Verification items for the finished model (mm, model axes). Face numbers are marked on the shaded views. A direction names the side the tool comes from. Coordinates: 2 decimals unless noted, no trailing zeros. Order: outer loops, then holes, each group sorted by start corner. A loop starts at its lowest first (then second) coordinate and runs counter-clockwise, first axis right, second up.
Q1. Draft check along X on the marked faces 1 and 2. Enter one of: pulls with the +X half, pulls with the -X half, needs draft (parallel to the pull), parting line crosses it, or undercut.
Q2. Depth check by flat-ended pin: P1, Ø2.5, axis at x = 23, y = 20.5, coming from the +Z side. Enter the tip coordinate at first touch or a pass-through.
Q3. Cross-section at D-D, the plane x = -14. Record the boundary of the cut face in (y, z), and give its area (3 significant figures).
Q4. Thickness scan on line 1 (X direction, y = 2, z = 4.2); line 2 (Y direction, x = 24, z = 3.1); line 3 (Y direction, x = -20, z = 3.05). Record the ranges inside material, lowest first.
Q5. Set-up check for the marked faces 3 and 4: record each of +Z, -Z, +X, -X, +Y, -Y from which the full face is reachable in a straight line by a thin tool's end or side.
Q6. Cross-section at A-A, the plane y = 20.5. Record the boundary of the cut face in (x, z).
Q7. Cross-section at B-B, the plane x = -23. Record the boundary of the cut face in (y, z), and give its area (3 significant figures).
Q8. Cross-section at C-C, the plane z = 4.2. Record the boundary of the cut face in (x, y).
from build123d import *

# Parameters (mm, degrees)
CROQUIS1_W              = 59
CROQUIS1_H              = 51
CROQUIS1_R              = 1.25
CROQUIS1_R_2            = 1.3
SALIENTE_EXTRUIR1_DEPTH = 5


with BuildPart() as part:
    # Croquis1 → Saliente-Extruir1 (new body)
    with BuildSketch(Plane.XY):
        with Locations((-0.238863052, -0.247607665)):
            Rectangle(CROQUIS1_W, CROQUIS1_H)
        with Locations((24.261136948, -17.747607665)):
            Circle(CROQUIS1_R, mode=Mode.SUBTRACT)
        with Locations((-18, 20.5)):
            Circle(CROQUIS1_R, mode=Mode.SUBTRACT)
        with Locations((18, 20.5)):
            Circle(CROQUIS1_R, mode=Mode.SUBTRACT)
        with Locations((-23, 20.5)):
            Circle(CROQUIS1_R_2, mode=Mode.SUBTRACT)
        with Locations((23, 20.5)):
            Circle(CROQUIS1_R_2, mode=Mode.SUBTRACT)
        with BuildLine():
            Line((-20.3, 5), (-20.3, -5))
            Line((-20.3, -5), (-15.007684576, -9.598280457))
            ThreePointArc((-15.007684576, -9.598280457), (-7, -12.591121267), (1.007684576, -9.598280457))
            Line((1.007684576, -9.598280457), (6.3, -5))
            Line((6.3, -5), (6.3, 5))
            Line((6.3, 5), (1.007684576, 9.598280457))
            ThreePointArc((1.007684576, 9.598280457), (-7, 12.591121267), (-15.007684576, 9.598280457))
            Line((-15.007684576, 9.598280457), (-20.3, 5))
        make_face(mode=Mode.SUBTRACT)
    extrude(amount=SALIENTE_EXTRUIR1_DEPTH)


solid = part.part
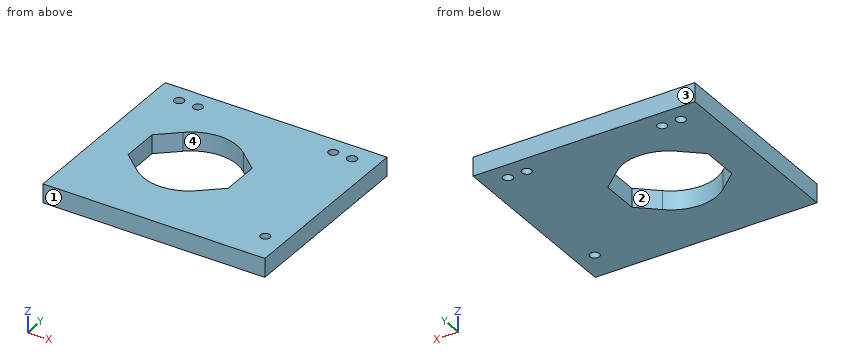
Check values:
1. face 1: needs draft
1. face 2: undercut
2. P1: passes through
3. outline: (-25.75, 0) - (-10.39, 0) - (-10.39, 5) - (-25.75, 5) - close; (10.39, 0) - (25.25, 0) - (25.25, 5) - (10.39, 5) - close
3. area: 151 mm2
4. line 1: x = -29.74 to -20.3, 6.3 to 29.26
4. line 2: y = -25.75 to -18.97, -16.53 to 19.67, 21.33 to 25.25
4. line 3: y = -25.75 to -5.26, 5.26 to 25.25
5. face 3: +Z, -Z, +X, -X, +Y
5. face 4: +Z, -Z
6. outline: (-29.74, 0) - (-24.3, 0) - (-24.3, 5) - (-29.74, 5) - close; (-21.7, 0) - (-19.25, 0) - (-19.25, 5) - (-21.7, 5) - close; (-16.75, 0) - (16.75, 0) - (16.75, 5) - (-16.75, 5) - close; (19.25, 0) - (21.7, 0) - (21.7, 5) - (19.25, 5) - close; (24.3, 0) - (29.26, 0) - (29.26, 5) - (24.3, 5) - close
7. outline: (-25.75, 0) - (19.2, 0) - (19.2, 5) - (-25.75, 5) - close; (21.8, 0) - (25.25, 0) - (25.25, 5) - (21.8, 5) - close
7. area: 242 mm2
8. outline: (-29.74, -25.75) - (29.26, -25.75) - (29.26, 25.25) - (-29.74, 25.25) - close; hole circle Ø2.6 at (-23, 20.5); hole (-20.3, -5) - (-15.01, -9.6) arc R12.21 ccw to (1.01, -9.6) - (6.3, -5) - (6.3, 5) - (1.01, 9.6) arc R12.21 ccw to (-15.01, 9.6) - (-20.3, 5) - close; hole circle Ø2.5 at (-18, 20.5); hole circle Ø2.5 at (18, 20.5); hole circle Ø2.6 at (23, 20.5); hole circle Ø2.5 at (24.26, -17.75)
